Build history of the part. All positions in model axes, mm. Coordinates: 2 decimals unless noted, no trailing zeros. Loops run counter-clockwise (first coordinate to the right, second up) from the corner with the lowest first, then second, coordinate; pieces in that order, holes last.
(1) Flat gauge pin, fed straight in: P1, Ø2, axis at x = -0.5, z = -7.5, coming from the +Y side. Where does the tip first touch, or does it go through?
(2) Slice it at A-A (y = 0). Give the cut face in (x, z).
(3) Wall check: L1, parallel to Z at x = -0.2, y = -0.3; L2, parallel to X at y = -0.75, z = 1.25; L3, parallel to Z at x = 1.1, y = -0.6. Give the ranges that are in metal, low to high.
(4) Two-plate mould, pull along Y, no slides. Class faces 1 (the face through (0, 0, -12)), 2 (the face through (0, 1, -6)), 3 (the face through (0, 0, 0.5)): pulls with the +Y half, pulls with the -Y half, needs draft (parallel to the pull), parting line crosses it, or undercut.
(5) Slice it at B-B (z = -2.75). Give the cut face in (x, y), and give its area (3 significant figures).
Autodesk Inventor part; units mm, degrees
ref_plane "YZ Plane" through (0, 0, 0) normal (1, 0, 0) x (0, 1, 0)
ref_plane "XZ Plane" through (0, 0, 0) normal (0, 1, 0) x (-1, 0, 0)
ref_plane "XY Plane" through (0, 0, 0) normal (0, 0, 1) x (1, 0, 0)
sketch "スケッチ1" plane through (0, 0, 0) normal (0, 0, 1) x (1, 0, 0)
  circle A0 centre (0, 0) radius 1.9
  dimension "d0" = 3.8
extrude "押し出し1" add sketch "スケッチ1" along normal blind 2
sketch "スケッチ2" plane through (0, 0, 0) normal (0, 0, -1) x (-1, 0, 0)
  circle A0 centre (0, 0) radius 1.9
  circle A1 centre (0, 0) radius 1
  dimension "d3" = 2
extrude "押し出し2" add sketch "スケッチ2" along normal blind 12 contours A1
sketch "スケッチ3" plane through (0, 0, 2) normal (0, 0, 1) x (1, 0, 0)
  circle A0 centre (0, 0) radius 1.9
  line L0 (0, 0.866) -> (0.75, 0.433)
  line L1 (0.75, 0.433) -> (0.75, -0.433)
  line L2 (0.75, -0.433) -> (0, -0.866)
  line L3 (0, -0.866) -> (-0.75, -0.433)
  line L4 (-0.75, -0.433) -> (-0.75, 0.433)
  line L5 (-0.75, 0.433) -> (0, 0.866)
  dimension "d6" = 0.75
extrude "押し出し3" cut sketch "スケッチ3" against normal blind 1.5 contours L0 L1 L2 L3 L4 L5
fillet "フィレット1" radius 0.5 2 edges at (-1.9, 0, 2) (-1.9, 0, 0)
fillet "フィレット2" radius 0.3 19 edges at (-0.375, 0.6495, 2) (-0.75, 0, 2) (-0.375, -0.6495, 2) (0.375, -0.6495, 2) (0.75, 0, 2) (0.375, 0.6495, 2) (-0.375, 0.6495, 0.5) (0.375, 0.6495, 0.5) (0, 0.866, 1.25) (-0.75, 0.433, 1.25) (-0.375, -0.6495, 0.5) (-0.75, -0.433, 1.25) (-0.75, 0, 0.5) (0.75, 0, 0.5) (0.75, 0.433, 1.25) (0.75, -0.433, 1.25) (0.375, -0.6495, 0.5) (0, -0.866, 1.25) (1, 0, -12)
thread "ねじ3"
Response values:
1. P1: stops at y = 1
2. outline: (-1.9, 0.5) arc R0.5 ccw to (-1.4, 0) - (-1, 0) - (-1, -11.7) arc R0.3 ccw to (-0.7, -12) - (0.7, -12) arc R0.3 ccw to (1, -11.7) - (1, 0) - (1.4, 0) arc R0.5 ccw to (1.9, 0.5) - (1.9, 1.5) arc R0.5 ccw to (1.4, 2) - (1.05, 2) arc R0.3 ccw to (0.75, 1.7) - (0.75, 0.8) arc R0.3 cw to (0.45, 0.5) - (-0.45, 0.5) arc R0.3 cw to (-0.75, 0.8) - (-0.75, 1.7) arc R0.3 ccw to (-1.05, 2) - (-1.4, 2) arc R0.5 ccw to (-1.9, 1.5) - close
3. L1: z = -12 to 0.5
3. L2: x = -1.75 to -0.2, 0.2 to 1.75
3. L3: z = 0 to 2
4. face 1: needs draft
4. face 2: parting line crosses it
4. face 3: undercut
5. outline: circle Ø2 at (0, 0)
5. area: 3.14 mm2
